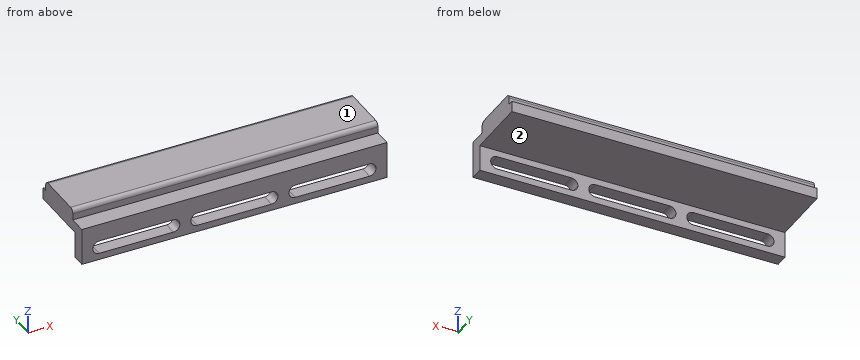
from build123d import *

# Parameters (mm, degrees)
F1_DEPTH = 70
F2_R     = 2
F4_DEPTH = 25


with BuildPart() as f1:
    # F0 (on Right) → F1 (new body, symmetric)
    with BuildSketch(Plane.YZ):
        Polygon((-20, 5), (-20, -12), (-14, -12), (-14, 0), (14.4, 0), (14.4, 5), (12, 5), (12, 10), (-12, 10), (-12, 5), align=None)
    extrude(amount=F1_DEPTH, both=True)

    # F2
    f2_edges = [f1.edges().sort_by_distance(p)[0] for p in [
        (0, -12, 10),
        (0, 12, 10),
    ]]
    fillet(f2_edges, radius=F2_R)

    # F3 (on face) → F4 (cut)
    with BuildSketch(Plane.XZ.offset(20)):
        with BuildLine():
            Line((-28, -3), (-62, -3))
            ThreePointArc((-62, -3), (-64.12132, -3.87868), (-65, -6))
            ThreePointArc((-65, -6), (-64.12132, -8.12132), (-62, -9))
            Line((-62, -9), (-28, -9))
            ThreePointArc((-28, -9), (-25.87868, -8.12132), (-25, -6))
            ThreePointArc((-25, -6), (-25.87868, -3.87868), (-28, -3))
        make_face()
        with BuildLine():
            Line((17, -3), (-17, -3))
            ThreePointArc((-17, -3), (-19.12132, -3.87868), (-20, -6))
            ThreePointArc((-20, -6), (-19.12132, -8.12132), (-17, -9))
            Line((-17, -9), (17, -9))
            ThreePointArc((17, -9), (19.12132, -8.12132), (20, -6))
            ThreePointArc((20, -6), (19.12132, -3.87868), (17, -3))
        make_face()
        with BuildLine():
            Line((62, -3), (28, -3))
            ThreePointArc((28, -3), (25.87868, -3.87868), (25, -6))
            ThreePointArc((25, -6), (25.87868, -8.12132), (28, -9))
            Line((28, -9), (62, -9))
            ThreePointArc((62, -9), (64.12132, -8.12132), (65, -6))
            ThreePointArc((65, -6), (64.12132, -3.87868), (62, -3))
        make_face()
    extrude(amount=-F4_DEPTH, mode=Mode.SUBTRACT)


solid = f1.part
Geometry check sheet. Reference: the model listing, model coordinates, mm. Face numbers are marked on the shaded views. A direction names the side the tool comes from. Round coordinates to 2 decimals unless told otherwise and drop trailing zeros. Loops run counter-clockwise (first coordinate to the right, second up) from the corner with the lowest first, then second, coordinate; pieces in that order, holes last.
Item 1: Gauge pin test, flat ends, axial feed: pin 1 (3.5 mm diameter, centred on x = -17.5, z = -3, fed in from +Y); pin 2 (1.2 mm diameter, centred on x = -1, y = 13, fed in from +Z); pin 3 (2.5 mm diameter, centred on x = 20.5, z = 7, fed in from +Y). Record the tip position at first contact, or that the pin passes through.
Item 2: Cross-section at D-D on y = -2. Record the boundary of the cut face in (x, z).
Item 3: Thickness scan on line 1 (X direction, y = -18, z = -7); line 2 (Z direction, x = -58.5, y = -15.5); line 3 (Z direction, x = -54.5, y = 10). Record the ranges inside material, lowest first.
Item 4: Access from +Z, -Z, +X, -X, +Y, -Y to the whole of each face (thin tool, end or side, straight path). Record for the marked faces 1 and 2.
Item 5: Cross-section at B-B on z = -7.25. Record the boundary of the cut face in (x, y), then the cut area to 3 significant figures.
Item 6: Cross-section at A-A on x = 59. Record the boundary of the cut face in (y, z), then the cut area to 3 significant figures.
Item 7: Cross-section at C-C on x = -23. Record the boundary of the cut face in (y, z), then the cut area to 3 significant figures.
Answer sheet:
1. pin 1: stops at y = -14
1. pin 2: stops at z = 5
1. pin 3: stops at y = 12
2. outline: (-70, 0) - (70, 0) - (70, 10) - (-70, 10) - close
3. line 1: x = -70 to -64.83, -25.17 to -19.83, 19.83 to 25.17, 64.83 to 70
3. line 2: z = -12 to -9, -3 to 5
3. line 3: z = 0 to 10
4. face 1: +Z, +X, -X, +Y, -Y
4. face 2: -Z, +X, -X, +Y
5. outline: (-70, -20) - (-64.73, -20) - (-64.73, -14) - (-70, -14) - close; (-25.27, -20) - (-19.73, -20) - (-19.73, -14) - (-25.27, -14) - close; (19.73, -20) - (25.27, -20) - (25.27, -14) - (19.73, -14) - close; (64.73, -20) - (70, -20) - (70, -14) - (64.73, -14) - close
5. area: 130 mm2
6. outline: (-20, -12) - (-14, -12) - (-14, -9) - (-20, -9) - close; (-20, -3) - (-14, -3) - (-14, 0) - (14.4, 0) - (14.4, 5) - (12, 5) - (12, 8) arc R2 ccw to (10, 10) - (-10, 10) arc R2 ccw to (-12, 8) - (-12, 5) - (-20, 5) - close
6. area: 326 mm2
7. outline: (-20, -12) - (-14, -12) - (-14, 0) - (14.4, 0) - (14.4, 5) - (12, 5) - (12, 8) arc R2 ccw to (10, 10) - (-10, 10) arc R2 ccw to (-12, 8) - (-12, 5) - (-20, 5) - close
7. area: 362 mm2
